Here's how the part is built. I have some questions about the finished solid (model axes, mm). Round coordinates to 2 decimals unless told otherwise and drop trailing zeros. Loops run counter-clockwise (first coordinate to the right, second up) from the corner with the lowest first, then second, coordinate; pieces in that order, holes last. Notation, with made-up numbers: M 9,79.5 L 17,79.5 A35 cw 17,115.5 Z; hole C -5.5,47.25 d5. An arc over 180 degrees is marked long. Answer as a JSON object with one key per item and string values.
from build123d import *

# Parameters (mm, degrees)
F0_R     = 1.75
F1_DEPTH = 5
F2_R     = 2
F2_W     = 65
F2_H     = 10
F3_DEPTH = 5.001
F5_DEPTH = 5


with BuildPart() as f1:
    # F0 (on Top) → F1 (new body)
    with BuildSketch(Plane.XY):
        Polygon((157.5, 107.5), (-157.5, 107.5), (-157.5, 62.5), (137.5, 62.5), (137.5, -62.5), (-157.5, -62.5), (-157.5, -107.5), (157.5, -107.5), (157.5, -62.5), (157.5, 62.5), align=None)
        with Locations((-95, -97.5)):
            Circle(F0_R, mode=Mode.SUBTRACT)
        with Locations((95, -97.5)):
            Circle(F0_R, mode=Mode.SUBTRACT)
        with Locations((-95, 97.5)):
            Circle(F0_R, mode=Mode.SUBTRACT)
        with Locations((95, 97.5)):
            Circle(F0_R, mode=Mode.SUBTRACT)
    extrude(amount=F1_DEPTH)

    # F2 (on face) → F3 (cut, through all)
    with BuildSketch(Plane.XY.offset(5)):
        with Locations((-154.5, -104.5)):
            Circle(F2_R)
        with Locations((154.5, 274.5)):
            Circle(F2_R)
        with Locations((-59.5786754345, 247.2672616252)):
            Circle(F2_R)
        with Locations((5, -102.5)):
            Rectangle(F2_W, F2_H)
        with Locations((154.5, -104.5)):
            Circle(F2_R)
        with Locations((-154.5, 104.5)):
            Circle(F2_R)
        with Locations((154.5, 104.5)):
            Circle(F2_R)
    extrude(amount=-F3_DEPTH, mode=Mode.SUBTRACT)

    # F4 (on face) → F5 (join, through all)
    with BuildSketch(Plane.XY.offset(5)):
        Polygon((-157.5, 62.5), (-157.5, 107.5), (157.5, 107.5), (157.5, -107.5), (37.5, -107.5), (37.5, -109.5), (159.5, -109.5), (159.5, 109.5), (-159.5, 109.5), (-159.5, 62.5), align=None)
        Polygon((-27.5, -107.5), (-157.5, -107.5), (-157.5, -62.5), (-159.5, -62.5), (-159.5, -109.5), (-27.5, -109.5), align=None)
    extrude(amount=-F5_DEPTH)


solid = f1.part
Item 1: I want a section at D-D on y = 6. List the corners of the cut face in (x, z) for me, plus the area to 3 significant figures.
Solution:
{"outline": "M 137.5,0 L 159.5,0 L 159.5,5 L 137.5,5 Z", "area": "110 mm2"}
Item 2: I want a section at A-A on x = -62. List the corners of the cut face in (y, z) for me.
Solution:
{"outline": "M -109.5,0 L -62.5,0 L -62.5,5 L -109.5,5 Z; M 62.5,0 L 109.5,0 L 109.5,5 L 62.5,5 Z"}
Item 3: If I drill on L1, parallel to X at y = 97.5, z = 2.85; L2, parallel to Y at x = -95, z = 1.8; L3, parallel to Y at x = 154.5, z = 3.3, over which ranges is the centre line in solid material (lowest first)? Write a range as from..to.
Solution:
{"L1": "x = -159.5..-96.75, -93.25..93.25, 96.75..159.5", "L2": "y = -109.5..-99.25, -95.75..-62.5, 62.5..95.75, 99.25..109.5", "L3": "y = -109.5..-106.5, -102.5..102.5, 106.5..109.5"}
Item 4: I want a section at C-C on x = 32. List the corners of the cut face in (y, z) for me, plus the area to 3 significant figures.
Solution:
{"outline": "M -97.5,0 L -62.5,0 L -62.5,5 L -97.5,5 Z; M 62.5,0 L 109.5,0 L 109.5,5 L 62.5,5 Z", "area": "410 mm2"}
Item 5: I want a section at B-B on z = 2.2. Count the separate pieces of the cut face and the enclosed holes in it, plus the area to 3 significant figures.
Solution:
{"separate pieces": "1", "enclosed holes": "8", "area": "31,900 mm2"}
Item 6: For P1, Ø4, axis at x = 95, y = 97.5, coming from the +Z side; P2, Ø2, axis at x = 95, y = -97.5, coming from the +Z side; P3, Ø2.5, axis at y = 30, z = 3, coming from the -X side, each with a flat end and sliding along its axis, tell me the tip position at first contact or that it passes through.
Solution:
{"P1": "stops at z = 5", "P2": "passes through", "P3": "stops at x = 137.5"}
